Input: part model. Units: mm. Frame: model coordinates. Round coordinates to 2 decimals unless told otherwise and drop trailing zeros. Loops run counter-clockwise (first coordinate to the right, second up) from the corner with the lowest first, then second, coordinate; pieces in that order, holes last.
1) First-contact query: pin 1 (2 mm diameter, centred on x = -0.5, z = 37, fed in from -Y); pin 2 (2 mm diameter, centred on x = 3, y = 4, fed in from -Z); pin 3 (6 mm diameter, centred on y = -4.5, z = 29.5, fed in from +X); pin 4 (5 mm diameter, centred on x = 1.5, y = -0.5, fed in from -Z) (1 decimal). Flat tips, straight axial feed; report the tip coordinate or a pass-through.
2) Draft query along X for faces 1 (the face through (0.62, -4.72, 37.95)), 2 (the face through (0.8, -6.3, 37.6)), 3 (the face through (4.73, 1.44, 7.79)). Return one class per face: pulls with the +X half, pulls with the -X half, needs draft (parallel to the pull), parting line crosses it, or undercut.
3) Ray query, line 1 along Y through (x, z) = (0.25, 52); line 2 along Y through (x, z) = (1, 58); line 3 along X through (y, z) = (-1.5, 72). Return the intervals inside material, ascending.
4) Section A-A, the plane y = 0. Return loops of the section in (x, z).
5) Section B-B, the plane x = 0. Return loops of the section in (y, z), and give its area (3 significant figures).
from build123d import *

# Parameters (mm, degrees)
SKETCH1_R           = 6.35
SKETCH1_R_2         = 4.7625
BOSS_EXTRUDE1_DEPTH = 76.2
CUT_EXTRUDE1_DEPTH  = 38.1
CUT_EXTRUDE3_DEPTH  = 38.1


with BuildPart() as part:
    # Sketch1 → Boss-Extrude1 (new body)
    with BuildSketch(Plane.XY):
        with Locations(Location((0, 0, 0), (0, 0, 180))):
            Circle(SKETCH1_R)
        with Locations(Location((0, 0, 0), (0, 0, 180))):
            Circle(SKETCH1_R_2, mode=Mode.SUBTRACT)
    extrude(amount=BOSS_EXTRUDE1_DEPTH)

    # Sketch2 → Cut-Extrude1 (cut, symmetric)
    with BuildSketch(Plane(origin=(0, 0, 0), x_dir=(0, 0, -1), z_dir=(1, 0, 0))):
        Polygon((-76.2, -6.35), (-68.867651581, 6.35), (-76.2, 6.35), align=None)
    extrude(amount=CUT_EXTRUDE1_DEPTH, both=True, mode=Mode.SUBTRACT)

    # Sketch3 → Cut-Extrude3 (cut, symmetric)
    with BuildSketch(Plane(origin=(0, 0, 0), x_dir=(0, 0, -1), z_dir=(1, 0, 0))):
        Polygon((-12.7, 6.35), (0, -6.35), (0, 6.35), align=None)
    extrude(amount=CUT_EXTRUDE3_DEPTH, both=True, mode=Mode.SUBTRACT)


solid = part.part
Final values:
1. pin 1: stops at y = -6.35
1. pin 2: stops at z = 9.52
1. pin 3: stops at x = 6.17
1. pin 4: passes through
2. face 1: undercut
2. face 2: parting line crosses it
2. face 3: needs draft
3. line 1: y = -6.35 to -4.76, 4.76 to 6.35
3. line 2: y = -6.27 to -4.66, 4.66 to 6.27
3. line 3: x = -6.17 to -4.52, 4.52 to 6.17
4. outline: (-6.35, 6.35) - (-4.76, 6.35) - (-4.76, 72.53) - (-6.35, 72.53) - close; (4.76, 6.35) - (6.35, 6.35) - (6.35, 72.53) - (4.76, 72.53) - close
5. outline: (-6.35, 0) - (-4.76, 1.59) - (-4.76, 75.28) - (-6.35, 76.2) - close; (4.76, 11.11) - (6.35, 12.7) - (6.35, 68.87) - (4.76, 69.78) - close
5. area: 210 mm2
